The model under review builds one solid part; all positions refer to its coordinate system, in mm. Coordinates: 2 decimals unless noted, no trailing zeros. Order: outer loops, then holes, each group sorted by start corner. A loop starts at its lowest first (then second) coordinate and runs counter-clockwise, first axis right, second up. Notation, with made-up numbers: M 76,66.5 L 115,66.5 A18 cw 115,93.5 Z; hole C 83,15.25 d6. An arc over 180 degrees is marked long. Answer in a Markdown table with one row per item.
from build123d import *

# Parameters (mm, degrees)
F0_W     = 127
F0_H     = 25.4
F1_DEPTH = 25.4
F2_DEPTH = 76.2
F3_R     = 25.39999
F4_R     = 25.39999


# Not quite as in the source:
# - a fillet or chamfer is up to 0.001 mm smaller than in the source, because OpenCascade refuses the exact size


with BuildPart() as f1:
    # F0 (on Front) → F1 (new body)
    with BuildSketch(Plane.XZ):
        with Locations((-27.0015653223, 9.674326013)):
            Rectangle(F0_W, F0_H)
        with BuildLine():
            Line((61.8984346777, 22.374326013), (36.4984346777, 22.374326013))
            Line((36.4984346777, 22.374326013), (36.4984346777, -3.025673987))
            ThreePointArc((36.4984346777, -3.025673987), (54.4589469199, 4.4138137708), (61.8984346777, 22.374326013))
        make_face()
    extrude(amount=F1_DEPTH)

    # F2 (add): a face of the model
    f2_faces = [f1.faces().sort_by_distance(p)[0] for p in [
        (-16.9176526174, -25.4, 9.9349632182),
    ]]
    extrude(f2_faces, amount=F2_DEPTH)

    # F3 (radius 25.4 in the source; OpenCascade refuses exactly that, so slightly less here)
    f3_edges = [f1.edges().sort_by_distance(p)[0] for p in [
        (-27.001565, -101.6, -3.025674),
    ]]
    fillet(f3_edges, radius=F3_R)

    # F4 (radius 25.4 in the source; OpenCascade refuses exactly that, so slightly less here)
    f4_edges = [f1.edges().sort_by_distance(p)[0] for p in [
        (-27.001565, 0, -3.025674),
    ]]
    fillet(f4_edges, radius=F4_R)


solid = f1.part
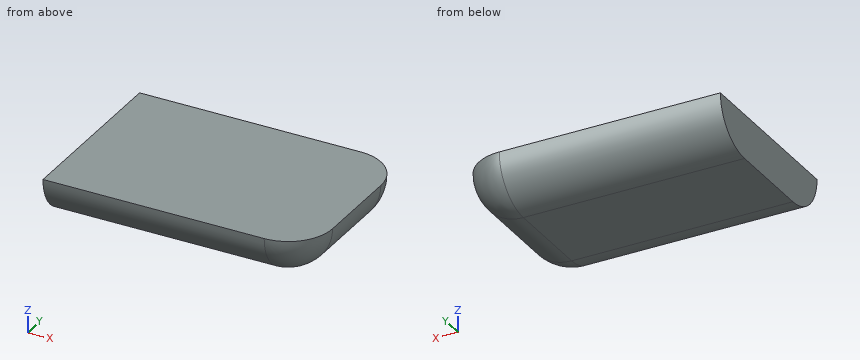
(1) Take a section at A-A (y = -70). Write out the cut boundary in (x, z), then the cut area to 3 significant figures.
Report:
| item | result |
|---|---|
| outline | M -90.5,-3.03 L 36.5,-3.03 A25.4 ccw 61.9,22.37 L -90.5,22.37 Z |
| area | 3,730 mm^2 |
(2) Insertion check: P1, Ø3, axis at y = -48, z = 17, coming from the +X side; P2, Ø3, axis at x = -39.5, z = 9, coming from the -Y side; P3, Ø6, axis at x = 31.5, y = -24, coming from the -Z side. Each pin has a flat end and moves straight along its axis. Give the tip position at first contact, or say it passes through.
Report:
| item | result |
|---|---|
| P1 | x = 61.6 |
| P2 | y = -98.65 |
| P3 | z = -3.03 |
(3) To check wall thickness, follow line 1 (Z direction, x = -78, y = -5.5); line 2 (X direction, y = -54.5, z = 7); line 3 (X direction, y = -55, z = 1.25). State the ranges of each line that lie inside material, in increasing order. Write a range as [from, to].
Report:
| item | result |
|---|---|
| line 1 | [6.59, 22.37] |
| line 2 | [-90.5, 56.72] |
| line 3 | [-90.5, 50.6] |
